Source: CAD feature listing. Evaluate the final solid. Frame: model axes, mm. A direction names the side the tool comes from. Coordinates: 2 decimals unless noted, no trailing zeros. Order: outer loops, then holes, each group sorted by start corner. A loop starts at its lowest first (then second) coordinate and runs counter-clockwise, first axis right, second up.
```python
from build123d import *

# Parameters (mm, degrees)
F0_W      = 127
F0_H      = 76.2
F1_DEPTH  = 4.572
F2_W      = 114.3
F2_H      = 76.2
F3_DEPTH  = 25.4
F4_W      = 63.5
F4_H      = 25.4
F4_W_2    = 12.7
F4_H_2    = 38.1
F4_R      = 38.6678322827
F5_DEPTH  = 25.4
F6_R      = 10.16
F7_R      = 2.54
F8_R      = 6.1321024484
F9_R      = 5.08
F10_R     = 10.16
F12_DEPTH = 5.08


with BuildPart() as f1:
    # F0 (on Top) → F1 (new body)
    with BuildSketch(Plane.XY):
        Rectangle(F0_W, F0_H)
    extrude(amount=F1_DEPTH)

    # F2 (on face) → F3 (join)
    with BuildSketch(Plane(origin=(0, 0, 0), x_dir=(1, 0, 0), z_dir=(0, 0, -1))):
        Rectangle(F2_W, F2_H)
    extrude(amount=F3_DEPTH)

    # F4 (on face) → F5 (cut)
    with BuildSketch(Plane(origin=(0, 0, -25.4), x_dir=(1, 0, 0), z_dir=(0, 0, -1))):
        with Locations((0, -25.4)):
            Rectangle(F4_W, F4_H)
        with Locations((-50.8, 19.05)):
            Rectangle(F4_W_2, F4_H_2)
        with Locations((50.8, 19.05)):
            Rectangle(F4_W_2, F4_H_2)
        with Locations((0, 38.1)):
            Circle(F4_R)
    extrude(amount=-F5_DEPTH, mode=Mode.SUBTRACT)

    # F6
    f6_edges = [f1.edges().sort_by_distance(p)[0] for p in [
        (-63.5, -38.1, 2.286),
    ]]
    fillet(f6_edges, radius=F6_R)

    # F7
    f7_edges = [f1.edges().sort_by_distance(p)[0] for p in [
        (-44.45, -38.1, -12.7),
        (38.667832, -38.1, -12.7),
        (-38.667832, -38.1, -12.7),
        (44.45, -38.1, -12.7),
        (57.15, 0, -12.7),
        (-57.15, 0, -12.7),
        (-31.75, 38.1, -12.7),
        (-57.15, 38.1, -12.7),
        (57.15, 38.1, -12.7),
        (31.75, 38.1, -12.7),
    ]]
    fillet(f7_edges, radius=F7_R)

    # F8
    f8_edges = [f1.edges().sort_by_distance(p)[0] for p in [
        (-44.45, 0, -12.7),
        (44.45, 0, -12.7),
        (-31.75, 12.7, -12.7),
        (31.75, 12.7, -12.7),
    ]]
    fillet(f8_edges, radius=F8_R)

    # F9
    f9_edges = [f1.edges().sort_by_distance(p)[0] for p in [
        (-63.5, 38.1, 2.286),
        (63.5, 38.1, 2.286),
    ]]
    fillet(f9_edges, radius=F9_R)

    # F10
    f10_edges = [f1.edges().sort_by_distance(p)[0] for p in [
        (63.5, -38.1, 2.286),
    ]]
    fillet(f10_edges, radius=F10_R)

    # F11 (on face) → F12 (cut)
    with BuildSketch(Plane(origin=(0, 0, 0), x_dir=(1, 0, 0), z_dir=(0, 0, -1))):
        with BuildLine():
            ThreePointArc((39.08503897, 37.0672740206), (39.0952697519, 37.5835919656), (39.0986802109, 38.1))
            Line((39.0986802109, 38.1), (38.6678322827, 38.1))
            Line((38.6678322827, 38.1), (-38.6678322827, 38.1))
            Line((-38.6678322827, 38.1), (-39.0986802109, 38.1))
            ThreePointArc((-39.0986802109, 38.1), (-39.0952697519, 37.5835919656), (-39.08503897, 37.0672740206))
            ThreePointArc((-39.08503897, 37.0672740206), (-38.7421543292, 36.4273480296), (-38.5943063027, 35.7165624699))
            ThreePointArc((-38.5943063027, 35.7165624699), (0, -0.5678322827), (38.5943063027, 35.7165624699))
            ThreePointArc((38.5943063027, 35.7165624699), (38.7421543292, 36.4273480296), (39.08503897, 37.0672740206))
        make_face()
    extrude(amount=-F12_DEPTH, mode=Mode.SUBTRACT)


solid = f1.part
```
1. Draft query along X for faces 6 (the face through (60.445, -35.203, 2.318)), 7 (the face through (30, 14.54, -12.52)), 8 (the face through (-56.426, 0.764, -12.522)). Return one class per face: released by +X, released by -X, zero draft, split by the parting line, or undercut.
Findings:
face 6: released by +X
face 7: undercut
face 8: released by -X
2. Pin query (flat end, axial travel): P1, Ø8.5, axis at y = 30.5, z = -14, coming from the -X side; P2, Ø12.5, axis at x = -10.5, z = -10, coming from the +Y side; P3, Ø1.2, axis at x = 52.5, z = -7.5, coming from the -Y side. Return the tip coordinate at first contact, or that it passes through.
Findings:
P1: stops at x = -57.15
P2: stops at y = 12.7
P3: stops at y = 0
3. Section query B-B on z = 1.25. Return loops of the section in (x, y).
Findings:
outline: (-63.5, -27.94) arc R10.16 ccw to (-53.34, -38.1) - (-39.1, -38.1) arc R39.1 cw to (-39.09, -37.07) arc R2.54 ccw to (-38.59, -35.72) arc R38.67 cw to (38.59, -35.72) arc R2.54 ccw to (39.09, -37.07) arc R39.1 cw to (39.1, -38.1) - (53.34, -38.1) arc R10.16 ccw to (63.5, -27.94) - (63.5, 33.02) arc R5.08 ccw to (58.42, 38.1) - (-58.42, 38.1) arc R5.08 ccw to (-63.5, 33.02) - close
4. Section query A-A on y = -20. Return loops of the section in (x, z).
Findings:
outline: (-63.5, 0) - (-44.45, 0) - (-44.45, -25.4) - (-34.17, -25.4) - (-34.17, 4.57) - (-63.5, 4.57) - close; (34.17, -25.4) - (44.45, -25.4) - (44.45, 0) - (63.5, 0) - (63.5, 4.57) - (34.17, 4.57) - close
5. Section query D-D on y = 15. Return loops of the section in (x, z), plus the area to 3 significant figures.
Findings:
outline: (-63.5, 0) - (-57.15, 0) - (-57.15, -25.4) - (-30.41, -25.4) - (-30.41, 0) - (30.41, 0) - (30.41, -25.4) - (57.15, -25.4) - (57.15, 0) - (63.5, 0) - (63.5, 4.57) - (-63.5, 4.57) - close
area: 1,940 mm2
6. Ray query, line 1 (X direction, y = 29.5, z = -9); line 2 (X direction, y = -14, z = -15.5); line 3 (Y direction, x = -52, z = -22). Return the intervals inside material, ascending.
Findings:
line 1: x = -57.15 to -31.75, 31.75 to 57.15
line 2: x = -44.45 to -30.24, 30.24 to 44.45
line 3: y = 0 to 38.1
7. Section query C-C on x = 0. Return loops of the section in (y, z).
Findings:
outline: (0.57, -25.4) - (12.7, -25.4) - (12.7, 0) - (38.1, 0) - (38.1, 4.57) - (0.57, 4.57) - close
8. Access query for faces 1 (the face through (-53, 0, -13)), 2 (the face through (-56.386, 37.376, -12.878)), 3 (the face through (46.29, -1.75, -12.52)), 4 (the face through (-29.91, 14.45, -12.52)), 5 (the face through (-57.15, 19, -13)). Directions: +Z, -Z, +X, -X, +Y, -Y. A direction counts if a zero-diameter tool reaches every point of the face in a straight line with its end or side. Return the directions, or none.
Findings:
face 1: -Z, -X, -Y
face 2: -Z, -X, +Y
face 3: -Z, +X, -Y
face 4: -Z, +Y
face 5: -Z, -X, +Y, -Y
